Autodesk Inventor part; units mm, degrees
ref_plane "Płaszczyzna konstrukcyjna4" through (64, 0, 8) normal (0, 0, 1) x (1, 0, 0)
ref_plane "Płaszczyzna konstrukcyjna5" through (64, 0, -8) normal (0, 0, 1) x (1, 0, 0)
ref_plane "Płaszczyzna konstrukcyjna7" through (7, 6, 0) normal (0, 1, 0) x (-1, 0, 0)
sketch "Szkic1" plane through (0, 0, 0) normal (0, 0, 1) x (1, 0, 0)
  line L0 (0, 6) -> (14, 6)
  line L1 (14, 6) -> (14, 0)
  line L2 (14, 6) -> (28, 10.5)
  line L3 (28, 10.5) -> (28, 0)
  line L4 (28, 10.5) -> (53.2879, 10.5)
  circle A0 centre (64, 0) radius 15
  line L5 (0, 6) -> (0, 0)
  line L6 (0, 0) -> (79, 0)
  dimension "d5" = 30
  dimension "d6" = 14
  dimension "d7" = 14
  dimension "d8" = 64
  dimension "d13" = 12
  dimension "d14" = 21
revolve "Obrót1" add sketch "Szkic1" angle 360 about axis through (0, 0, 0) along (1, 0, 0) picked at (60.2352, 8.4613) contours L0 L1 L6 L5 | L2 L3 L6 L1 | L4 A0 L6 L3 | A0 L6
ref_plane "Płaszczyzna konstrukcyjna1" through (64, 0, -15) normal (0, 0, 1) x (1, 0, 0)
ref_plane "Płaszczyzna konstrukcyjna3" through (64, 0, 0) normal (0, 0, 1) x (1, 0, 0)
ref_plane "Płaszczyzna konstrukcyjna2" through (64, 0, 15) normal (0, 0, 1) x (1, 0, 0)
ref_plane "Płaszczyzna konstrukcyjna4" through (64, 0, 8) normal (0, 0, 1) x (1, 0, 0)
ref_plane "Płaszczyzna konstrukcyjna5" through (64, 0, -8) normal (0, 0, 1) x (1, 0, 0)
sketch "Szkic2" plane through (64, 0, -8) normal (0, 0, 1) x (1, 0, 0)
  line L0 (18, 16) -> (-68, 16)
  line L1 (-68, 16) -> (-68, -17)
  line L2 (-68, -17) -> (18, -17)
  line L3 (18, -17) -> (18, 16)
  point P0 (-64, 0)
extrude "Wyciągnięcie proste1" cut sketch "Szkic2" against normal blind 10
sketch "Szkic3" plane through (64, 0, 8) normal (0, 0, 1) x (1, 0, 0)
  line L0 (20, 22) -> (-75, 22)
  line L1 (-75, 22) -> (-75, -17)
  line L2 (-75, -17) -> (20, -17)
  line L3 (20, -17) -> (20, 22)
  point P0 (-64, 0)
extrude "Wyciągnięcie proste2" cut sketch "Szkic3" along normal blind 10
sketch "Szkic4" plane through (64, 0, 8) normal (0, 0, 1) x (1, 0, 0)
  arc A0 (-10.7121, -10.5) -> (-10.7121, 10.5) centre (0, 0) ccw
  circle A1 centre (0, 0) radius 6
  point P0 (-64, 0)
  dimension "d19" = 12
extrude "Wyciągnięcie proste3" cut sketch "Szkic4" against normal up to surface (16 mm away)
ref_plane "Płaszczyzna konstrukcyjna6" through (7, 6, 0) normal (0, 1, 0) x (-1, 0, 0)
sketch "Szkic5" plane through (7, 6, 0) normal (0, 1, 0) x (-1, 0, 0)
  line L0 (7, 6) -> (7, -6)
  line L1 (7, -6) -> (-7, -6)
  line L2 (-7, 6) -> (-7, -6)
  line L3 (7, 6) -> (-7, 6)
  line L4 (7, -6) -> (-3, -6)
  line L5 (-3, -6) -> (-3, 6)
  line L6 (-3, 6) -> (7, 6)
  line L7 (7, 6) -> (7, -6)
  point P0 (7, 0)
  point P1 (-3, -6)
  dimension "d22" = 10
extrude "Wyciągnięcie proste4" cut sketch "Szkic5" against normal blind 3 contours L0 L1 L5 L3
ref_plane "Płaszczyzna konstrukcyjna7" through (7, 6, 0) normal (0, 1, 0) x (-1, 0, 0)
ref_plane "Płaszczyzna konstrukcyjna8" through (7, -6, 0) normal (0, 1, 0) x (-1, 0, 0)
sketch "Szkic6" plane through (7, -6, 0) normal (0, 1, 0) x (-1, 0, 0)
  point P0 (7, 0)
sketch "Szkic7" plane through (7, -6, 0) normal (0, 1, 0) x (-1, 0, 0)
  line L0 (7, 6) -> (-3, 6)
  line L1 (-3, 6) -> (-3, -6)
  line L2 (-3, -6) -> (7, -6)
  line L3 (7, -6) -> (7, 6)
  point P0 (7, 0)
extrude "Wyciągnięcie proste5" cut sketch "Szkic7" along normal blind 3
sketch "Szkic8" plane through (7, 6, 0) normal (0, 1, 0) x (-1, 0, 0)
  circle A0 centre (2, 0) radius 2.5
  line L0 (7, 5.1962) -> (7, -5.1962)
  point P0 (7, 0)
  dimension "d28" = 5
  dimension "d29" = 5
extrude "Wyciągnięcie proste6" cut sketch "Szkic8" against normal through all
properties part number "Bartosz_Zukowski_walek_04_10"
Here's how the part is built. I have some questions about the finished solid (model axes, mm). A direction names the side the tool comes from. Coordinates: 2 decimals unless noted, no trailing zeros. Loops run counter-clockwise (first coordinate to the right, second up) from the corner with the lowest first, then second, coordinate; pieces in that order, holes last. Notation, with made-up numbers: M 17,35 L 36,35 A32 ccw 36,73 Z; hole C 88,40.5 d2. An arc over 180 degrees is marked long. One line per item, written item: value.
1. Imagine slicing it at C-C (z = 0). List the corners of the cut face in (x, y) for me.
Geometry says:
outline: M 0,-3 L 2.5,-3 L 2.5,3 L 0,3 Z; M 7.5,-3 L 10,-3 L 10,-6 L 14,-6 L 28,-10.5 L 53.29,-10.5 A15 ccw long 53.29,10.5 L 28,10.5 L 14,6 L 10,6 L 10,3 L 7.5,3 Z; hole C 64,0 d12
2. Will these pins go through, and if not, where does the flat tip stop? pin 1 Ø8 at (x, z) = (2.5, 2) entering from -Y; pin 2 Ø3 at (x, z) = (5.5, 1.5) entering from +Y; pin 3 Ø3 at (y, z) = (-11, -0.5) entering from +X; pin 4 Ø4.5 at (x, z) = (5, 0) entering from -Y.
Geometry says:
pin 1: stops at y = -3
pin 2: stops at y = 3
pin 3: stops at x = 75.6
pin 4: passes through
3. Thinking about a two-plate mould opening in X: for faces 1 (the cylindrical face through (58, 0, 0)), 2 (the cylindrical face through (2.615, 0.042, 0.751)), 3 (the flat face through (0, 0, 0)), 4 (the flat face through (6.2, -3, 2.4)), which applies, +X half, -X half, draft (parallel to the pull), parting line (faces both ways), or undercut?
Geometry says:
face 1: undercut
face 2: undercut
face 3: -X half
face 4: draft
4. Imagine slicing it at B-B (x = 5). List the corners of the cut face in (y, z) for me.
Geometry says:
outline: M -3,-5.2 A6 ccw 3,-5.2 L 3,-2.5 L -3,-2.5 Z; M -3,2.5 L 3,2.5 L 3,5.2 A6 ccw -3,5.2 Z
5. Imagine slicing it at D-D (x = 64). List the corners of the cut face in (y, z) for me, and give its area (3 significant figures).
Geometry says:
outline: M -12.69,-8 L -6,-8 L -6,8 L -12.69,8 A15 ccw Z; M 6,-8 L 12.69,-8 A15 ccw 12.69,8 L 6,8 Z
area: 264 mm2
6. Imagine slicing it at A-A (y = 0). List the corners of the cut face in (x, z) for me.
Geometry says:
outline: M 0,-6 L 14,-6 L 20.22,-8 L 58,-8 L 58,8 L 20.22,8 L 14,6 L 0,6 Z; M 70,-8 L 76.69,-8 A15 ccw 76.69,8 L 70,8 Z; hole C 5,0 d5
7. Please list where these lines run through material, in increasing order: probe 1 along Y at (x, z) = (8, 4); probe 2 along Y at (x, z) = (69, 1.5); probe 3 along Y at (x, z) = (64, -2).
Geometry says:
probe 1: y = -3 to 3
probe 2: y = -14.06 to -3.32, 3.32 to 14.06
probe 3: y = -14.87 to -6, 6 to 14.87
8. On a 3-axis mill with a long thin cutter (end or side, diameter ignored), from which of +Z, -Z, +X, -X, +Y, -Y can I reach the whole of each face in a straight line? I mean faces 5 (the flat face through (6.2, 3, 2.4)), 6 (the cylindrical face through (8.654, -1.301, -5.857)), 7 (the cylindrical face through (40.8, -10.5, 0.1)). Say none if no direction works.
Geometry says:
face 5: +Z, -Z, -X, +Y
face 6: -X
face 7: -X, -Y
